Autodesk Inventor part; units mm, degrees
ref_plane "YZ Plane" through (0, 0, 0) normal (1, 0, 0) x (0, 1, 0)
ref_plane "XZ Plane" through (0, 0, 0) normal (0, 1, 0) x (-1, 0, 0)
ref_plane "XY Plane" through (0, 0, 0) normal (0, 0, 1) x (1, 0, 0)
sketch "Sketch1" plane through (0, 0, 0) normal (0, 0, 1) x (1, 0, 0)
  line L0 (-0.0175, -6.5307) -> (-20.2143, -18.1913)
  line L1 (-23.3893, -12.6921) -> (-0.0175, 0.8017)
  line L2 (-0.0175, 0.8017) -> (23.3544, -12.6921)
  line L3 (20.1794, -18.1913) -> (-0.0175, -6.5307)
  line L4 (-0.0175, 0.8017) -> (-0.0175, -6.5307) construction
  line L5 (-20.2143, -18.1913) -> (-23.3893, -12.6921)
  line L6 (20.1794, -18.1913) -> (23.3544, -12.6921)
  dimension "d4" = 120
  dimension "d5" = 6.35
  dimension "d6" = 26.9875
extrude "Extrusion1" add sketch "Sketch1" along normal blind 25.4
hole "Hole1" at (9.1809, -11.8413, 12.7) direction (0.5, 0.8660254, 0) diameter 6.756 end through all
hole "Hole2" at (-9.2158, -11.8413, 12.7) direction (-0.5, 0.8660254, 0) diameter 6.756 end through all
fillet "Fillet1" radius 2 2 edges at (-0.0175, -6.5307, 12.7) (-0.0175, 0.8017, 12.7)
fillet "Fillet2" radius 0.25 20 edges at (-23.3893, -12.6921, 12.7) (-20.2143, -18.1913, 12.7) (20.1794, -18.1913, 12.7) (23.3544, -12.6921, 12.7) (-0.0175, 0.4923, 25.4) (-12.2034, -6.2339, 25.4) (12.1685, -6.2339, 25.4) (-0.0175, -6.8401, 25.4) (-10.6159, -12.6497, 25.4) (10.581, -12.6497, 25.4) (-21.8018, -15.4417, 25.4) (21.7669, -15.4417, 25.4) (-21.8018, -15.4417, 0) (-0.0175, 0.4923, 0) (12.1685, -6.2339, 0) (-12.2034, -6.2339, 0) (-0.0175, -6.8401, 0) (10.581, -12.6497, 0) (-10.6159, -12.6497, 0) (21.7669, -15.4417, 0)
chamfer "Chamfer1" distance 0.25 angle 45 4 edges at (-9.2158, -11.8413, 16.078) (9.1809, -11.8413, 16.078) (-12.3908, -6.3421, 16.078) (12.3559, -6.3421, 16.078)
properties part number "drive_frame_bracket" material "Aluminum-6061"
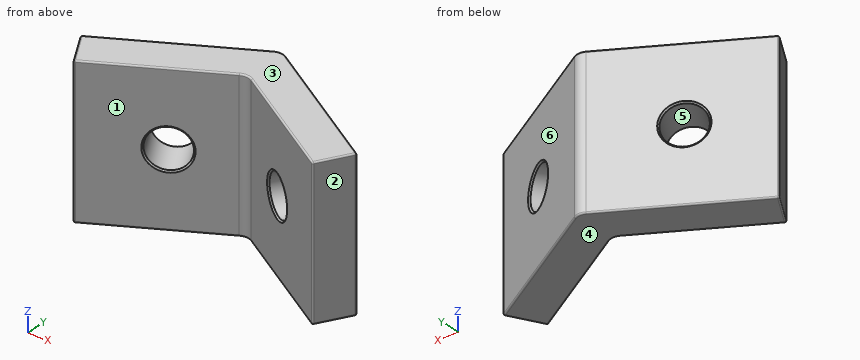
The listing builds one solid part. Answer for the finished solid, in the listing's coordinates (mm). Face numbers are marked on the shaded views. A direction names the side the tool comes from. Give positions to 0.01 mm unless a question says otherwise; leave off trailing zeros. Order: outer loops, then holes, each group sorted by start corner. A loop starts at its lowest first (then second) coordinate and runs counter-clockwise, first axis right, second up. Notation, with made-up numbers: (54, 48) - (61, 48) arc R20 cw to (61, 83) - close; hole circle Ø11 at (-32, 57.25). An arc over 180 degrees is marked (long way). Answer as CSV lines item,"result".
Q1. Each of these flat-tipped pins is pushed along its axis until it touches: pin 1 Ø5 at (y, z) = (-4.5, 21) entering from +X; pin 2 Ø4 at (x, z) = (12, 15.5) entering from +Y; pin 3 Ø6 at (x, z) = (15, 19.5) entering from +Y. Where does it stop, or does it pass through?
Answer key:
pin 1,"stops at x = 13.5"
pin 2,"stops at y = -4.98"
pin 3,"stops at y = -6.14"
Q2. Determine the mould class of the marked faces 3, 4, 5 and 6 for opening direction Z: pulls with the +Z half, pulls with the -Z half, needs draft (parallel to the pull), parting line crosses it, or undercut.
Answer key:
face 3,"pulls with the +Z half"
face 4,"pulls with the -Z half"
face 5,"undercut"
face 6,"needs draft"
Q3. Straight lines are drawn through the part: L1, parallel to X at y = -13, z = 7.5; L2, parallel to X at y = -7.75, z = 11.25; L3, parallel to Y at x = -11.5, z = 18. For each, find the intervals that lie inside material, in ascending order.
Answer key:
L1,"x = -23.21 to -11.22, 11.19 to 23.18"
L2,"x = -8.05 to -2.13, 2.09 to 8.02"
L3,"y = -13.16 to -5.83"
Q4. A cutting plane is placed at A-A, the plane z = 5.5. Determine the outline of the cut face in (x, y), and give its area (3 significant figures).
Answer key:
outline,"(-23.26, -12.91) - (-20.34, -17.97) arc R0.25 ccw to (-20, -18.07) - (-1.02, -7.11) arc R2 cw to (0.98, -7.11) - (19.96, -18.07) arc R0.25 ccw to (20.3, -17.97) - (23.23, -12.91) arc R0.25 ccw to (23.14, -12.57) - (0.98, 0.22) arc R2 ccw to (-1.02, 0.22) - (-23.17, -12.57) arc R0.25 ccw to start"
area,"319 mm^2"
Q5. Which of the six approach directions +Z, -Z, +X, -X, +Y, -Y give full straight-line access (tool end or side, diameter ignored) to the marked faces 1 and 2?
Answer key:
face 1,"+Z, -Z, -Y"
face 2,"+Z, -Z, +X, -Y"
